from build123d import *

# Parameters (mm, degrees)
SKETCH1_W           = 23.75
SKETCH1_H           = 7.5
BOSS_EXTRUDE1_DEPTH = 8
FILLET1_R           = 3.75
FILLET2_R           = 3.75
CUT_EXTRUDE13_DEPTH = 27.159367347
CUT_EXTRUDE14_DEPTH = 10


with BuildPart() as part:
    # Sketch1 → Boss-Extrude1 (new body)
    with BuildSketch(Plane.XY):
        with Locations((11.875, 3.75)):
            Rectangle(SKETCH1_W, SKETCH1_H)
    extrude(amount=BOSS_EXTRUDE1_DEPTH)

    # Fillet1
    fillet1_edges = [part.edges().sort_by_distance(p)[0] for p in [
        (23.75, 0, 4),
        (23.75, 7.5, 4),
    ]]
    fillet(fillet1_edges, radius=FILLET1_R - 0.0001)  # a hair under: the kernel refuses the full size

    # Fillet2
    fillet2_edges = [part.edges().sort_by_distance(p)[0] for p in [
        (0, 0, 4),
        (0, 7.5, 4),
    ]]
    fillet(fillet2_edges, radius=FILLET2_R - 0.0001)  # a hair under: the kernel refuses the full size

    # Sketch17 → Cut-Extrude13 (cut, through all)
    with BuildSketch(Plane.XY.offset(8)):
        Polygon((21, 6.25), (20, 6.25), (20, 3.75), (22.5, 3.75), (22.5, 4.75), (21, 4.75), align=None)
        Polygon((20, 3.75), (20, 6.25), (19, 6.25), (19, 4.75), (17.5, 4.75), (17.5, 2.75), (19, 2.75), (19, 1.25), (20, 1.25), align=None)
        Polygon((22.5, 3.75), (20, 3.75), (20, 1.25), (21, 1.25), (21, 2.75), (22.5, 2.75), align=None)
    cut_extrude13 = extrude(amount=-CUT_EXTRUDE13_DEPTH, mode=Mode.SUBTRACT)

    # Mirror4: Cut-Extrude13 across plane
    add(cut_extrude13.mirror(Plane(origin=(11.875, 0, 0), x_dir=(0, 0, 1), z_dir=(1, 0, 0))), mode=Mode.SUBTRACT)

    # Sketch18 → Cut-Extrude14 (cut)
    with BuildSketch(Plane(origin=(0, 7.5, 0), x_dir=(1, 0, 0), z_dir=(0, 1, 0))):
        Polygon((14.375, -4), (11.875, -4), (11.875, -6.5), (12.875, -6.5), (12.875, -5), (14.375, -5), align=None)
        Polygon((11.875, -4), (13.90625, -3), (12.875, -3), (12.875, -1.5), (11.875, -1.5), align=None)
        Polygon((14.375, -3), (13.90625, -3), (11.875, -4), (14.375, -4), align=None)
        Polygon((9.84375, -5), (11.875, -4), (11.875, -1.5), (10.875, -1.5), (10.875, -3), (9.375, -3), (9.375, -5), align=None)
        Polygon((11.875, -6.5), (11.875, -4), (9.84375, -5), (10.875, -5), (10.875, -6.5), align=None)
    extrude(amount=-CUT_EXTRUDE14_DEPTH, mode=Mode.SUBTRACT)


solid = part.part
The model under review builds one solid part; all positions refer to its coordinate system, in mm. A direction names the side the tool comes from. Round coordinates to 2 decimals unless told otherwise and drop trailing zeros. Order: outer loops, then holes, each group sorted by start corner. A loop starts at its lowest first (then second) coordinate and runs counter-clockwise, first axis right, second up. Notation, with made-up numbers: (20, 34) -> (28, 34) arc R20 ccw to (28, 60) -> close; hole circle Ø3 at (71.25, -14.5). An arc over 180 degrees is marked (long way). Write item = value, one per line. Start each with the question number.
Item 1: Consider section B-B on y = 2. Write out the cut boundary in (x, z) (3 decimals), plus the area to 3 significant figures.
Item 2: For faces 1 (the face through (10, 0, 6)), 2 (the face through (14.375, 4, 4)), 3 (the face through (2, 4.75, 4)), list the 3-axis set-ups (+Z, -Z, +X, -X, +Y, -Y) from which the entire face can be reached by the end or side of a thin tool; tool diameter is ignored.
Item 3: For line 1 along Y through (x, z) = (20, 2.25); line 2 along Z through (x, y) = (10.5, 6); line 3 along X through (y, z) = (2, 4.25) (3 decimals), list the stretches that pass through material, from the lowest coordinate up.
Item 4: Clearance check with flat-ended pins moving along their axes: pin 1 Ø1.2 at (y, z) = (2, 3) entering from -X; pin 2 Ø2 at (y, z) = (5.5, 4) entering from +X; pin 3 Ø2 at (y, z) = (5, 4) entering from -X. State where each tip first meets the part, or that it passes through.
Item 5: Mouldability with a two-part tool opening along Y and no side actions: class faces 4 (the face through (10, 4, 5)), 5 (the face through (18, 2.75, 4)), 6 (the face through (10, 7.5, 6)) as released by +Y, released by -Y, zero draft, split by the parting line, or undercut.
Item 6: Consider section A-A on x = 10.5. Write out the cut boundary in (y, z), plus the area to 3 significant figures.
Item 7: Consider section C-C on z = 2.5. Count the separate pieces of the cut face and the enclosed holes in it, plus the area to 3 significant figures.
Conclusion:
q1.outline = (0.433, 0) -> (2.75, 0) -> (2.75, 8) -> (0.433, 8) -> close; (4.75, 0) -> (19, 0) -> (19, 8) -> (4.75, 8) -> close; (21, 0) -> (23.317, 0) -> (23.317, 8) -> (21, 8) -> close; hole (9.375, 3) -> (10.875, 3) -> (10.875, 1.5) -> (12.875, 1.5) -> (12.875, 3) -> (14.375, 3) -> (14.375, 5) -> (12.875, 5) -> (12.875, 6.5) -> (10.875, 6.5) -> (10.875, 5) -> (9.375, 5) -> close
q1.area = 135 mm2
q2.face_1 = +Z, -Z, +X, -X, -Y
q2.face_2 = +Y, -Y
q2.face_3 = +Z, -Z
q3.line_1 = 0 to 1.25, 6.25 to 7.5
q3.line_2 = 0 to 3, 5 to 8
q3.line_3 = 0.433 to 2.75, 4.75 to 9.375, 14.375 to 19, 21 to 23.317
q4.pin_1 = 0.18
q4.pin_2 = 23.67
q4.pin_3 = 0.01
q5.face_4 = zero draft
q5.face_5 = undercut
q5.face_6 = released by +Y
q6.outline = (0, 0) -> (7.5, 0) -> (7.5, 3) -> (0, 3) -> close; (0, 5) -> (7.5, 5) -> (7.5, 8) -> (0, 8) -> close
q6.area = 45.0 mm2
q7.separate_pieces = 2
q7.enclosed_holes = 2
q7.area = 119 mm2
